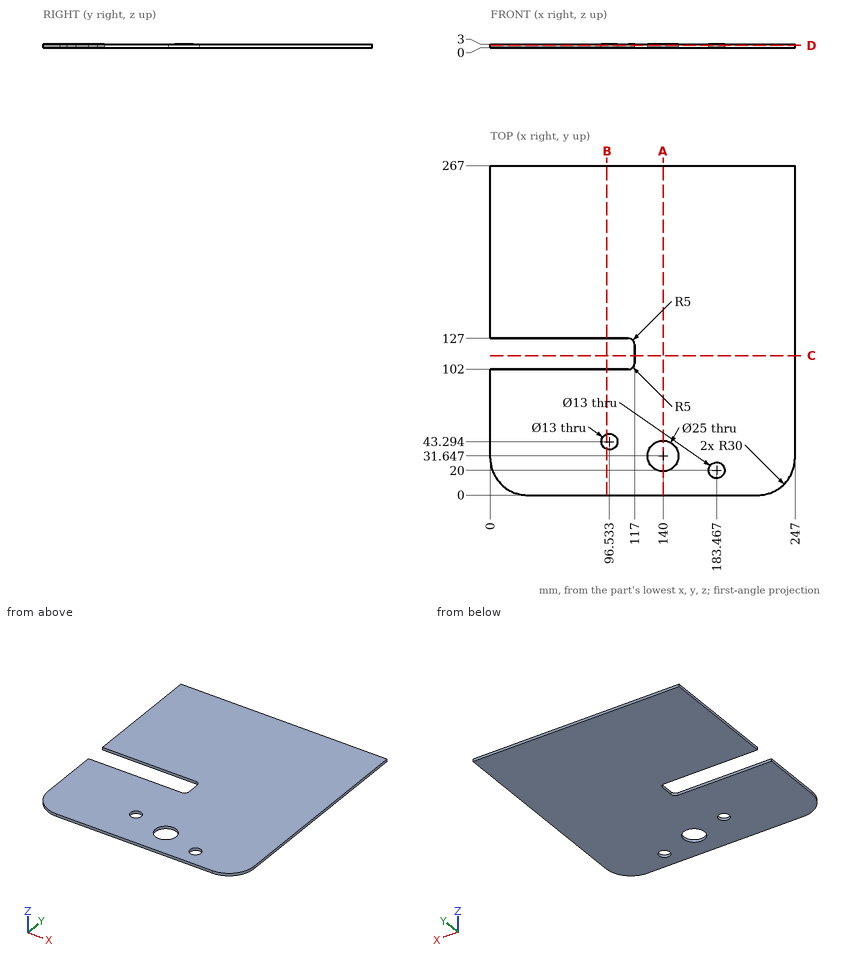
Print and shaded views of the part. All mm, measured from the part's lowest x, y and z. Coordinates: 2 decimals unless noted, no trailing zeros. Loops run counter-clockwise (first coordinate to the right, second up) from the corner with the lowest first, then second, coordinate; pieces in that order, holes last. Notation, with made-up numbers: (70, -29.75) -> (123, -29.75) arc R25 ccw to (123, -9.75) -> close; hole circle Ø11 at (-40, 63). An arc over 180 degrees is marked (long way). Use a Markdown table: item, result. Add a question column.
Item 1: Band-saw the part on C-C on y = 113. Write the cut outline in (x, z), plus the area to 3 significant figures.
Item 2: Band-saw the part on B-B on x = 94.5. Write the cut outline in (y, z), plus the area to 3 significant figures.
Item 3: Probe probe 1 along Y at (x, z) = (97, 0.3); probe 2 along Y at (x, z) = (140, 0.8); probe 3 along Y at (x, z) = (111, 1.05). List the from-to ranges inside material, lowest first.
Item 4: Band-saw the part on D-D on z = 1.85. Write the cut outline in (x, y), plus the area to 3 significant figures.
Item 5: Band-saw the part on A-A on x = 140. Write the cut outline in (y, z).
Geometry says:
| question | item | result |
|---|---|---|
| 1 | outline | (117, 0) -> (247, 0) -> (247, 3) -> (117, 3) -> close |
| 1 | area | 390 mm² |
| 2 | outline | (0, 0) -> (37.12, 0) -> (37.12, 3) -> (0, 3) -> close; (49.47, 0) -> (102, 0) -> (102, 3) -> (49.47, 3) -> close; (127, 0) -> (267, 0) -> (267, 3) -> (127, 3) -> close |
| 2 | area | 689 mm² |
| 3 | probe 1 | 0 to 36.81, 49.78 to 102, 127 to 267 |
| 3 | probe 2 | 0 to 19.15, 44.15 to 267 |
| 3 | probe 3 | 0 to 102, 127 to 267 |
| 4 | outline | (0, 30) arc R30 ccw to (30, 0) -> (217, 0) arc R30 ccw to (247, 30) -> (247, 267) -> (0, 267) -> (0, 127) -> (112, 127) arc R5 cw to (117, 122) -> (117, 107) arc R5 cw to (112, 102) -> (0, 102) -> close; hole circle Ø13 at (96.53, 43.29); hole circle Ø25 at (140, 31.65); hole circle Ø13 at (183.47, 20) |
| 4 | area | 61,900 mm² |
| 5 | outline | (0, 0) -> (19.15, 0) -> (19.15, 3) -> (0, 3) -> close; (44.15, 0) -> (267, 0) -> (267, 3) -> (44.15, 3) -> close |
